Input: dimensioned drawing with shaded views. Units: mm. Origin: part minimum x, y, z. Coordinates: 2 decimals unless noted, no trailing zeros. Loops run counter-clockwise (first coordinate to the right, second up) from the corner with the lowest first, then second, coordinate; pieces in that order, holes last.
Item 1: Pull-direction query (X, two-part tool) for the marked faces 1, 2 and 3; classes: released by +X, released by -X, zero draft, split by the parting line, or undercut.
Item 2: Section A-A on x = 19.05. Return loops of the section in (y, z).
Item 3: Ray query, line 1 along Y through (x, z) = (19.05, 4.1); line 2 along X through (y, z) = (18, 5.25); line 3 along Y through (x, z) = (22, 2.15) (1 decimal). Return the intervals inside material, ascending.
Item 4: Section C-C on z = 0.5. Give the number of separate pieces and of enclosed holes in the cut face, and give its area (3 significant figures).
Item 5: Section D-D on y = 5. Return loops of the section in (x, z), and give its area (3 significant figures).
Item 6: Contact query for flat-ended pins moving along their axis: P1, Ø1, axis at x = 5.5, z = 2, coming from the +Y side; P2, Ø1, axis at x = 6, z = 2, coming from the -Y side (1 decimal); P3, Ø16.5, axis at x = 19.05, y = 19.05, coming from the +Z side. Output: stop coordinate, or through.
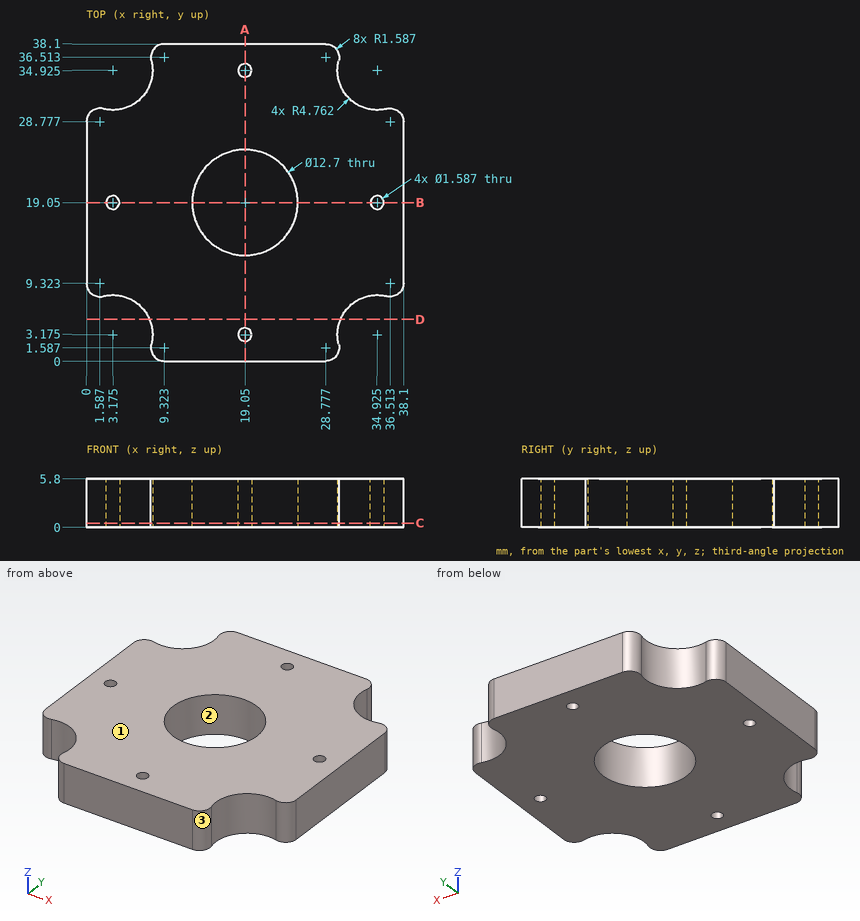
Results found:
1. face 1: zero draft
1. face 2: undercut
1. face 3: released by +X
2. outline: (0, 0) - (2.38, 0) - (2.38, 5.8) - (0, 5.8) - close; (3.97, 0) - (12.7, 0) - (12.7, 5.8) - (3.97, 5.8) - close; (25.4, 0) - (34.13, 0) - (34.13, 5.8) - (25.4, 5.8) - close; (35.72, 0) - (38.1, 0) - (38.1, 5.8) - (35.72, 5.8) - close
3. line 1: y = 0 to 2.38, 3.97 to 12.7, 25.4 to 34.13, 35.72 to 38.1
3. line 2: x = 0 to 12.79, 25.31 to 38.1
3. line 3: y = 0 to 13.4, 24.7 to 38.1
4. separate pieces: 1
4. enclosed holes: 5
4. area: 1,080 mm2
5. outline: (7.57, 0) - (30.53, 0) - (30.53, 5.8) - (7.57, 5.8) - close
5. area: 133 mm2
6. P1: stops at y = 31.09
6. P2: stops at y = 6.6
6. P3: stops at z = 5.8
